Job drawing, mm, ordinate dimensions from the low corner. One solid piece. A direction names the side the tool comes from. Give positions to 0.01 mm unless a question says otherwise; leave off trailing zeros. Order: outer loops, then holes, each group sorted by start corner. A loop starts at its lowest first (then second) coordinate and runs counter-clockwise, first axis right, second up. Notation, with made-up numbers: (74, 55.25) - (113, 55.25) arc R23 ccw to (113, 92.25) - close; hole circle Ø4 at (44, 57). An arc over 180 degrees is marked (long way). One line per item, written item: value.
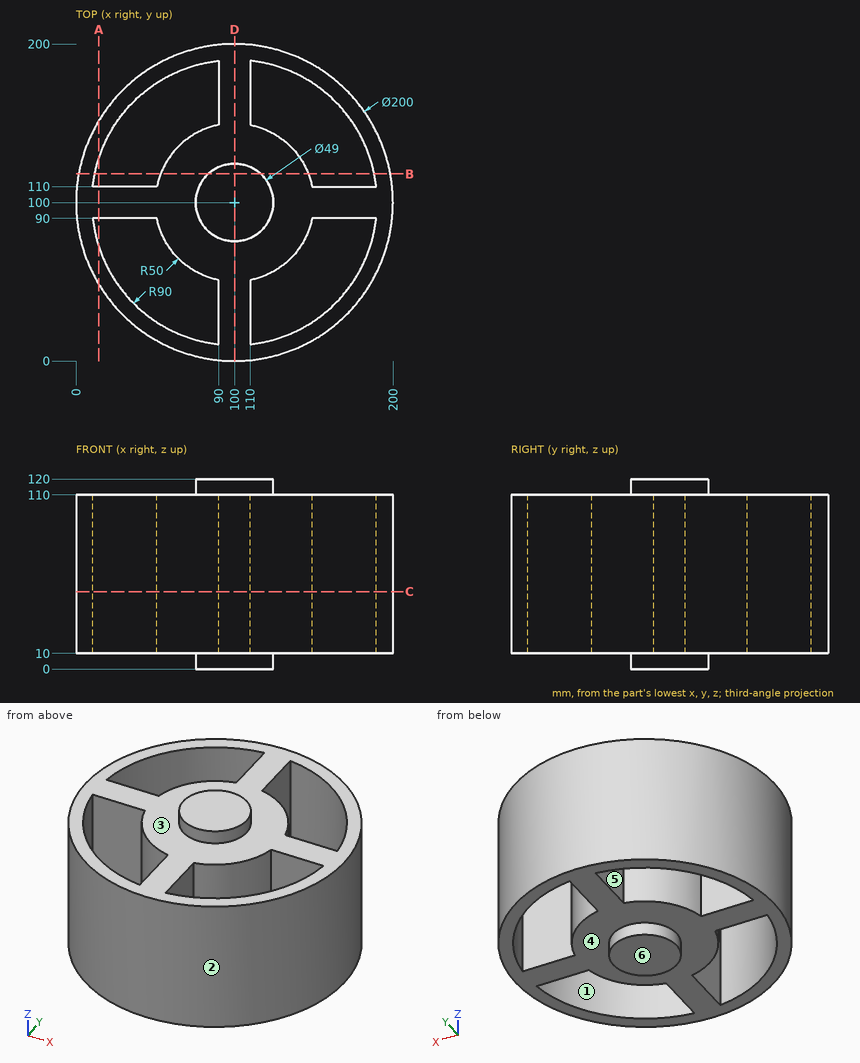
1) Slice it at D-D on x = 100. Write the cut outline in (y, z), then the cut area to 3 significant figures.
Answer:
outline: (0, 10) - (75.5, 10) - (75.5, 0) - (124.5, 0) - (124.5, 10) - (200, 10) - (200, 110) - (124.5, 110) - (124.5, 120) - (75.5, 120) - (75.5, 110) - (0, 110) - close
area: 21,000 mm2
2) Two-plate mould, pull along Y, no slides. Class the marked faces 1, 2 and 3: pulls with the +Y half, pulls with the -Y half, needs draft (parallel to the pull), parting line crosses it, or undercut.
Answer:
face 1: undercut
face 2: parting line crosses it
face 3: needs draft
3) Which spindle directions (+Z, -Z, +X, -X, +Y, -Y) get a long thin tool onto all of the face, cutting with end or side? Do the marked faces 4, 5 and 6. Say none if no direction does.
Answer:
face 4: -Z
face 5: +Z, -Z
face 6: -Z, +X, -X, +Y, -Y
4) Wall check: line 1 along Y through (x, z) = (76, 84); line 2 along X through (y, z) = (112, 79); line 3 along Y through (x, z) = (154, 49). Give the ranges that are in metal, low to high. Write a range as [from, to].
Answer:
line 1: y = [2.92, 13.26], [56.14, 143.86], [186.74, 197.08]
line 2: x = [0.72, 10.8], [51.46, 148.54], [189.2, 199.28]
line 3: y = [15.83, 28], [90, 110], [172, 184.17]
5) Slice it at A-A on x = 14.5. Write the cut outline in (y, z), then the cut area to 3 significant figures.
Answer:
outline: (48.14, 10) - (71.9, 10) - (71.9, 110) - (48.14, 110) - close; (90, 10) - (110, 10) - (110, 110) - (90, 110) - close; (128.1, 10) - (151.86, 10) - (151.86, 110) - (128.1, 110) - close
area: 6,750 mm2
6) Slice it at C-C on z = 49. Write the cut outline in (x, y).
Answer:
outline: circle Ø200 at (100, 100); hole (10.56, 90) arc R90 ccw to (90, 10.56) - (90, 51.01) arc R50 cw to (51.01, 90) - close; hole (10.56, 110) - (51.01, 110) arc R50 cw to (90, 148.99) - (90, 189.44) arc R90 ccw to start; hole (110, 10.56) arc R90 ccw to (189.44, 90) - (148.99, 90) arc R50 cw to (110, 51.01) - close; hole (110, 148.99) arc R50 cw to (148.99, 110) - (189.44, 110) arc R90 ccw to (110, 189.44) - close
7) Drop flat-ended pins along their axis: P1, Ø2, axis at y = 83, z = 77, coming from the +X side; P2, Ø4, axis at y = 27.5, z = 74.5, coming from the +X side; P3, Ø20, axis at y = 27.5, z = 39, coming from the +X side. Give the stop position or say it passes through.
Answer:
P1: stops at x = 198.71
P2: stops at x = 170.92
P3: stops at x = 178.06
8) Slice it at B-B on y = 118. Write the cut outline in (x, z), then the cut area to 3 significant figures.
Answer:
outline: (1.63, 10) - (11.82, 10) - (11.82, 110) - (1.63, 110) - close; (53.35, 10) - (83.38, 10) - (83.38, 0) - (116.62, 0) - (116.62, 10) - (146.65, 10) - (146.65, 110) - (116.62, 110) - (116.62, 120) - (83.38, 120) - (83.38, 110) - (53.35, 110) - close; (188.18, 10) - (198.37, 10) - (198.37, 110) - (188.18, 110) - close
area: 12,000 mm2
